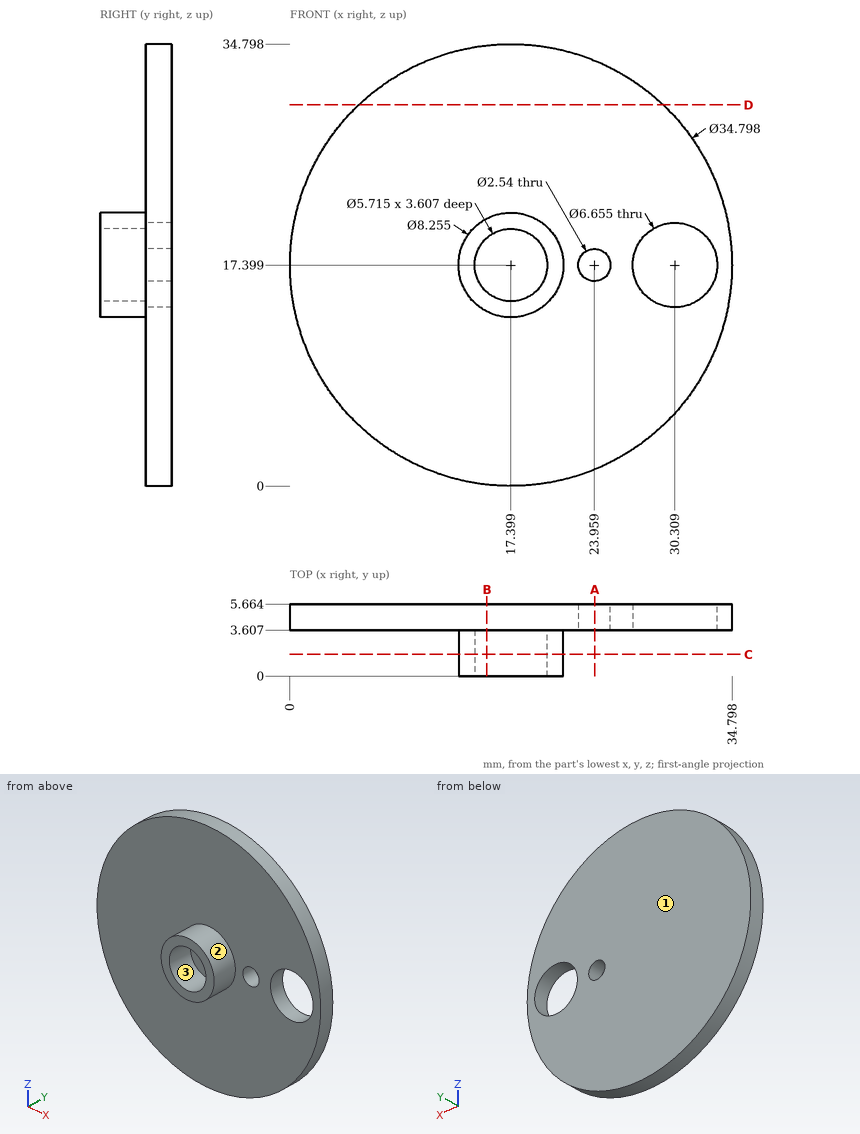
Geometry check sheet. Reference: drawing and pictorial views, mm from the part's lowest x, y, z. Round coordinates to 2 decimals unless told otherwise and drop trailing zeros. Order: outer loops, then holes, each group sorted by start corner. A loop starts at its lowest first (then second) coordinate and runs counter-clockwise, first axis right, second up. Notation, with made-up numbers: (-31, -33.75) - (-14, -33.75) arc R17 ccw to (-14, -29.75) - close; hole circle Ø4 at (-18.5, 43.25). An arc over 180 degrees is marked (long way). Write item = value, one per line.
Q1. Draft check along Z on the marked faces 1, 2 and 3. Enter one of: pulls with the +Z half, pulls with the -Z half, needs draft (parallel to the pull), parting line crosses it, or undercut.
Computed:
face_1 = needs draft
face_2 = parting line crosses it
face_3 = undercut
Q2. Go/stop test with flat-tipped pins: pin 1 (5 mm diameter, centred on x = 7.5, z = 3.5, fed in from -Y); pin 2 (2 mm diameter, centred on x = 19.5, y = 2.5, fed in from +Z); pin 3 (3 mm diameter, centred on y = 2.5, z = 20, fed in from +X) (1 decimal). Record where each tip stops, or that it passes through.
Computed:
pin_1 = 3.61
pin_2 = 21.38
pin_3 = 34.7
Q3. Section check B-B (x = 15.5). Record the boundary of the cut face in (y, z) (1 decimal).
Computed:
outline = (0, 13.7) - (3.6, 13.7) - (3.6, 0.1) - (5.7, 0.1) - (5.7, 34.7) - (3.6, 34.7) - (3.6, 21.1) - (0, 21.1) - (0, 19.5) - (3.6, 19.5) - (3.6, 15.3) - (0, 15.3) - close
Q4. Section check A-A (x = 24). Record the boundary of the cut face in (y, z) (1 decimal).
Computed:
outline = (3.6, 1.3) - (5.7, 1.3) - (5.7, 16.1) - (3.6, 16.1) - close; (3.6, 18.7) - (5.7, 18.7) - (5.7, 33.5) - (3.6, 33.5) - close
Q5. Thickness scan on line 1 along Y through (x, z) = (6, 27) (1 decimal); line 2 along Z through (x, y) = (17.5, 0.5) (1 decimal). Record the ranges inside material, lowest first.
Computed:
line_1 = 3.6 to 5.7
line_2 = 13.3 to 14.5, 20.3 to 21.5
Q6. Section check D-D (z = 30). Record the boundary of the cut face in (x, y) (1 decimal).
Computed:
outline = (5.4, 3.6) - (29.4, 3.6) - (29.4, 5.7) - (5.4, 5.7) - close
Q7. Section check C-C (y = 1.7). Record the boundary of the cut face in (x, z) (1 decimal).
Computed:
outline = circle Ø8.3 at (17.4, 17.4); hole circle Ø5.7 at (17.4, 17.4)
